Geometry: final body of the model. Coordinates: model frame, mm. Coordinates: 2 decimals unless noted, no trailing zeros. Order: outer loops, then holes, each group sorted by start corner. A loop starts at its lowest first (then second) coordinate and runs counter-clockwise, first axis right, second up. Notation, with made-up numbers: M -3.5,18 L 38.5,18 A14 ccw 38.5,32 Z; hole C -0.5,8.25 d5. An arc over 180 degrees is marked long. Write item = value, one per line.
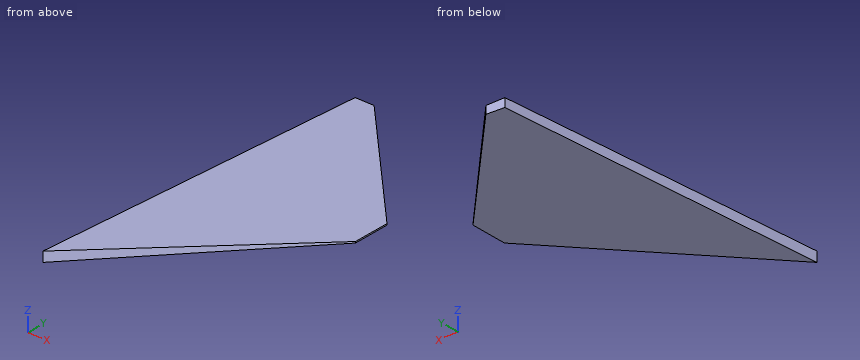
from build123d import *

# Parameters (mm, degrees)
BOSS_EXTRUDE1_DEPTH     = 508
CUT_EXTRUDE3_DEPTH      = 558.14262793
CUT_EXTRUDE3_DEPTH_BACK = 558.14262793


with BuildPart() as part:
    # Sketch1 → Boss-Extrude1 (new body)
    with BuildSketch(Plane(origin=(0, 0, 0), x_dir=(1, 0, 0), z_dir=(0, 1, 0))):
        Polygon((0, -3.937193282), (0, 9.270806718), (228.6, 2.666806718), (228.6, 0.888806718), align=None)
    extrude(amount=BOSS_EXTRUDE1_DEPTH)

    # Sketch3 → Cut-Extrude3 (cut, two sides: drawn at the far end of the back side and taken through both)
    with BuildSketch(Plane.XY.offset(-CUT_EXTRUDE3_DEPTH_BACK)):
        Polygon((228.6, 0), (0, 0), (151.300007346, 151.300007346), (228.6, 228.6), align=None)
        Polygon((228.6, 508), (228.6, 279.4), (58.436980759, 463.596176947), (33.036980759, 463.596176947), (0, 0), (0, 508), align=None)
    extrude(amount=CUT_EXTRUDE3_DEPTH + CUT_EXTRUDE3_DEPTH_BACK, mode=Mode.SUBTRACT)


solid = part.part
1) Line query: L1, parallel to Z at x = 30, y = 32; L2, parallel to Z at x = 32, y = 43.5; L3, parallel to Y at x = 102, z = -2.25. Output: solid intervals per line, ascending.
Numbers:
L1 = -8.4 to 3.3
L2 = -8.35 to 3.26
L3 = 102 to 416.44
2) Section C-C, the plane y = 189. Return loops of the section in (x, z).
Numbers:
outline = M 13.47,-8.88 L 189,-3.81 L 189,-0.05 L 13.47,3.65 Z
3) Section B-B, the plane x = 204.5. Return loops of the section in (y, z), and give its area (3 significant figures).
Numbers:
outline = M 204.5,-3.36 L 305.49,-3.36 L 305.49,-0.38 L 204.5,-0.38 Z
area = 301 mm²
4) Section A-A, the plane z = -5. Return loops of the section in (x, y).
Numbers:
outline = M 0,0 L 147.84,147.84 L 147.84,366.82 L 58.44,463.6 L 33.04,463.6 Z
5) Pin query (flat end, axial travel): pin 1 (2 mm diameter, centred on x = 183.5, y = 280, fed in from +Z); pin 2 (4 mm diameter, centred on y = 179, z = -2.5, fed in from -X); pin 3 (2 mm diameter, centred on x = 40.5, y = 213, fed in from -Z). Return the tip coordinate at first contact, or that it passes through.
Numbers:
pin_1 = 0.08
pin_2 = 12.61
pin_3 = -8.13
